Here's how the part is built. I have some questions about the finished solid (model axes, mm). A direction names the side the tool comes from. Round coordinates to 2 decimals unless told otherwise and drop trailing zeros. Order: outer loops, then holes, each group sorted by start corner. A loop starts at its lowest first (then second) coordinate and runs counter-clockwise, first axis right, second up.
```python
from build123d import *

# Parameters (mm, degrees)
SALIENTE_EXTRUIR1_DEPTH = 40
CORTAR_EXTRUIR1_DEPTH   = 35
SALIENTE_EXTRUIR2_DEPTH = 40


with BuildPart() as part:
    # Croquis1 → Saliente-Extruir1 (new body)
    with BuildSketch(Plane(origin=(0, 0, 0), x_dir=(1, 0, 0), z_dir=(0, 1, 0))):
        Polygon((14, -14), (14, 14), (-14, 14), (-74.822534414, 14), (-74.822534414, -14), (-14, -14), (-14, -54), (14, -54), align=None)
    extrude(amount=SALIENTE_EXTRUIR1_DEPTH)

    # Croquis2 → Cortar-Extruir1 (cut)
    with BuildSketch(Plane(origin=(0, 40, 0), x_dir=(1, 0, 0), z_dir=(0, 1, 0))):
        Polygon((9, 9), (-9, 9), (-74.822534414, 9), (-74.822534414, -9), (-9, -9), (-9, -54), (9, -54), (9, -9), align=None)
    extrude(amount=-CORTAR_EXTRUIR1_DEPTH, mode=Mode.SUBTRACT)

    # Croquis3 → Saliente-Extruir2 (add)
    with BuildSketch(Plane(origin=(0, 40, 0), x_dir=(1, 0, 0), z_dir=(0, 1, 0))):
        Polygon((-34, -14), (-14, -34), (-14, -14), align=None)
        Polygon((-34, -9), (-34, -4), (-26, -9), align=None)
        Polygon((-34, 4), (-26, 9), (-34, 9), align=None)
    extrude(amount=-SALIENTE_EXTRUIR2_DEPTH)


solid = part.part
```
1) If we section it at C-C (x = 1): Write out the boundary of the cut face in (y, z).
2) I need wall thicknesses on line 1 (X direction, y = 20.5, z = 13); line 2 (Z direction, x = -54, y = 35). Which ranges of each line are inside material? Lowest first, please.
3) If we section it at A-A (z = 35): Write out the boundary of the cut face in (x, y).
4) If we section it at B-B (y = 29): Write out the boundary of the cut face in (x, z).
5) We'd pull the mould along Z, two halves only. Please class faces 6 (the flat face through (-74.823, 20, -10)), 7 (the flat face through (-18, 23, 9)), 8 (the flat face through (-24, 20, 24)): +Z half, -Z half, draft (parallel to the pull), parting line (faces both ways), or undercut.
6) If we section it at D-D (y = 4): Write out the boundary of the cut face in (x, z), plus the area to 3 significant figures.
7) For faces 1 (the flat face through (-55, 20, 14)), 2 (the flat face through (-17, 40, -10)), 3 (the flat face through (9, 23, 23)), 4 (the flat face through (-8, 23, -9)), 5 (the flat face through (-34, 23, -7)), which set-ups out of +Z, -Z, +X, -X, +Y, -Y let a thin tool reach every point of the face, with its end or its side?
8) I'm going to push flat-ended pins straight in: pin 1 (16 mm diameter, centred on y = 20.5, z = 41.5, fed in from -X); pin 2 (1.5 mm diameter, centred on y = 23.5, z = -6, fed in from -X); pin 3 (8 mm diameter, centred on y = 7, z = 33, fed in from -X). Where does each tip first touch, or does it pass through?
Solutions:
1. outline: (0, -14) - (40, -14) - (40, -9) - (5, -9) - (5, 54) - (0, 54) - close
2. line 1: x = -74.82 to -9, 9 to 14
2. line 2: z = -14 to -9, 9 to 14
3. outline: (-14, 0) - (14, 0) - (14, 40) - (9, 40) - (9, 5) - (-9, 5) - (-9, 40) - (-14, 40) - close
4. outline: (-74.82, -14) - (14, -14) - (14, 54) - (9, 54) - (9, -9) - (-26, -9) - (-34, -4) - (-34, -9) - (-74.82, -9) - close; (-74.82, 9) - (-34, 9) - (-34, 4) - (-26, 9) - (-9, 9) - (-9, 54) - (-14, 54) - (-14, 34) - (-34, 14) - (-74.82, 14) - close
5. face 6: draft
5. face 7: undercut
5. face 8: +Z half
6. outline: (-74.82, -14) - (14, -14) - (14, 54) - (-14, 54) - (-14, 34) - (-34, 14) - (-74.82, 14) - close
6. area: 3,810 mm2
7. face 1: +Z, -X, +Y, -Y
7. face 2: +Z, -Z, +X, -X, +Y
7. face 3: +Z, +Y
7. face 4: +Y
7. face 5: -X, +Y
8. pin 1: stops at x = -14.5
8. pin 2: stops at x = -34
8. pin 3: stops at x = -19
